Source: CAD feature listing. Evaluate the final solid. Frame: model axes, mm. A direction names the side the tool comes from. Round coordinates to 2 decimals unless told otherwise and drop trailing zeros. Loops run counter-clockwise (first coordinate to the right, second up) from the corner with the lowest first, then second, coordinate; pieces in that order, holes last. Notation, with made-up numbers: (2.5, 9.5) - (10.5, 9.5) arc R20 cw to (10.5, 19.5) - close; hole circle Ø7 at (70, 57). An arc over 180 degrees is marked (long way). One line per question, with ' | ' between items. Start each with the question number.
1. Ray query, line 1 (Z direction, x = -3.5, y = 5.75); line 2 (X direction, y = 0.75, z = -4.75); line 3 (X direction, y = -6.25, z = 1.5). Return the intervals inside material, ascending.
2. Pin query (flat end, axial travel): pin 1 (1.5 mm diameter, centred on x = 5.5, z = 1, fed in from -Y); pin 2 (2 mm diameter, centred on x = -8, z = 0.5, fed in from +Y). Return the tip coordinate at first contact, or that it passes through.
3. Cut plane B-B (z = 1.5). Return loops of the section in (x, y).
4. Cut plane C-C (y = 7.25). Return loops of the section in (x, z), then the cut area to 3 significant figures.
5. Access query for faces 1 (the flat face through (0, -7, 0)), 2 (the flat face through (-6, -4, 3.302)), 3 (the flat face through (-3.33, 5.81, 1.63)). Directions: +Z, -Z, +X, -X, +Y, -Y. A direction counts if a zero-diameter tool reaches every point of the face in a straight line with its end or side. Return the directions, or none.
6. Cut plane D-D (x = 6). Return loops of the section in (y, z).
7. Mould query, pull axis X, two halves, no side actions, for faces 4 (the flat face through (6, 4, 0)), 5 (the flat face through (2.487, 6.104, 1.628)), 6 (the flat face through (-6.53, -0.9, 1.63)), 7 (the flat face through (-3.366, -5.791, 1.628)). Classes: pulls with the +X half, pulls with the -X half, needs draft (parallel to the pull), parting line crosses it, or undercut.
```python
from build123d import *

# Parameters (mm, degrees)
F1_DEPTH    = 3.302
F2_DEPTH    = 6.35
F3_T1_DEPTH = 4.6338919233
F4_T1_DEPTH = 4.4582047696


# Not quite as in the source:
# - a fillet or chamfer that OpenCascade refuses, or shapes differently, is made with other operations: its cross-section is extruded or revolved along the edge and cut away or added


with BuildPart() as f1:
    # F0 (on Top) → F1 (new body)
    with BuildSketch(Plane.XY):
        with BuildLine():
            Line((0.8864303251, 2.1758656964), (4.1494522244, 10.1854037464))
            ThreePointArc((4.1494522244, 10.1854037464), (-0.7354841661, 10.9735803766), (-5.4715498037, 9.5405736717))
            Line((-5.4715498037, 9.5405736717), (-1.1688645655, 2.0381133132))
            ThreePointArc((-1.1688645655, 2.0381133132), (-0.157118442, 2.3442406116), (0.8864303251, 2.1758656964))
        make_face()
    extrude(amount=F1_DEPTH)



with BuildPart() as f1b:
    # F0 (on Top) → F1, piece 2 (new body)
    with BuildSketch(Plane.XY):
        with BuildLine():
            Line((-2.3275701308, -0.320261668), (-10.8955445044, -1.4991708351))
            ThreePointArc((-10.8955445044, -1.4991708351), (-9.1356572935, -6.1237381602), (-5.5266042645, -9.5087879639))
            Line((-5.5266042645, -9.5087879639), (-1.1806256223, -2.0313230639))
            ThreePointArc((-1.1806256223, -2.0313230639), (-1.9516127013, -1.3081888679), (-2.3275701308, -0.320261668))
        make_face()
    extrude(amount=F1_DEPTH)


with BuildPart() as f1c:
    # F0 (on Top) → F1, piece 3 (new body)
    with BuildSketch(Plane.XY):
        with BuildLine():
            ThreePointArc((6.74609228, -8.6862329113), (9.8711414597, -4.8498422164), (10.9981540682, -0.0317857078))
            Line((10.9981540682, -0.0317857078), (2.3494901878, -0.0067902494))
            ThreePointArc((2.3494901878, -0.0067902494), (2.1087311432, -1.0360517437), (1.4411398058, -1.8556040284))
            Line((1.4411398058, -1.8556040284), (6.74609228, -8.6862329113))
        make_face()
    extrude(amount=F1_DEPTH)


with BuildPart() as f1_1:
    add(f1.part)

    add(f1b.part)  # F2 merges F1b

    add(f1c.part)  # F2 merges F1c
    # F0 (on Top) → F2 (join)
    with BuildSketch(Plane.XY):
        with BuildLine():
            ThreePointArc((10.9981540682, -0.0317857078), (10.9981885171, -0.0158928705), (10.9982, 0))
            ThreePointArc((10.9982, 0), (9.1267986911, 6.136933183), (4.1494522244, 10.1854037464))
            Line((4.1494522244, 10.1854037464), (0.8864303251, 2.1758656964))
            ThreePointArc((0.8864303251, 2.1758656964), (1.9497202747, 1.3110076661), (2.3495, 0))
            ThreePointArc((2.3495, 0), (2.3494975469, -0.0033951282), (2.3494901878, -0.0067902494))
            Line((2.3494901878, -0.0067902494), (10.9981540682, -0.0317857078))
        make_face()
        with BuildLine():
            Line((0.8864303251, 2.1758656964), (4.1494522244, 10.1854037464))
            ThreePointArc((4.1494522244, 10.1854037464), (-0.7354841661, 10.9735803766), (-5.4715498037, 9.5405736717))
            Line((-5.4715498037, 9.5405736717), (-1.1688645655, 2.0381133132))
            ThreePointArc((-1.1688645655, 2.0381133132), (-0.157118442, 2.3442406116), (0.8864303251, 2.1758656964))
        make_face()
        with BuildLine():
            ThreePointArc((6.74609228, -8.6862329113), (9.8711414597, -4.8498422164), (10.9981540682, -0.0317857078))
            Line((10.9981540682, -0.0317857078), (2.3494901878, -0.0067902494))
            ThreePointArc((2.3494901878, -0.0067902494), (2.1087311432, -1.0360517437), (1.4411398058, -1.8556040284))
            Line((1.4411398058, -1.8556040284), (6.74609228, -8.6862329113))
        make_face()
        with BuildLine():
            Line((-1.1688645655, 2.0381133132), (-5.4715498037, 9.5405736717))
            ThreePointArc((-5.4715498037, 9.5405736717), (-9.8711414597, 4.8498422164), (-10.8955445044, -1.4991708351))
            Line((-10.8955445044, -1.4991708351), (-2.3275701308, -0.320261668))
            ThreePointArc((-2.3275701308, -0.320261668), (-2.1087311432, 1.0360517437), (-1.1688645655, 2.0381133132))
        make_face()
        with BuildLine():
            ThreePointArc((-5.5266042645, -9.5087879639), (0.7354841661, -10.9735803766), (6.74609228, -8.6862329113))
            Line((6.74609228, -8.6862329113), (1.4411398058, -1.8556040284))
            ThreePointArc((1.4411398058, -1.8556040284), (0.157118442, -2.3442406116), (-1.1806256223, -2.0313230639))
            Line((-1.1806256223, -2.0313230639), (-5.5266042645, -9.5087879639))
        make_face()
        with BuildLine():
            Line((-2.3275701308, -0.320261668), (-10.8955445044, -1.4991708351))
            ThreePointArc((-10.8955445044, -1.4991708351), (-9.1356572935, -6.1237381602), (-5.5266042645, -9.5087879639))
            Line((-5.5266042645, -9.5087879639), (-1.1806256223, -2.0313230639))
            ThreePointArc((-1.1806256223, -2.0313230639), (-1.9516127013, -1.3081888679), (-2.3275701308, -0.320261668))
        make_face()
    extrude(amount=-F2_DEPTH)

    # F3: fillet of radius 0.508 on 6 edges, made by hand

    # F3_s2 → F3_t1 (cut)
    with BuildSketch(Plane.XY):
        with BuildLine():
            ThreePointArc((3.9531481969, 9.7035483908), (3.9459668292, 10.1036299064), (3.6513440541, 10.3743958782))
            ThreePointArc((3.6513440541, 10.3743958782), (3.901542663, 10.2829163222), (4.1494522244, 10.1854037464))
            Line((4.1494522244, 10.1854037464), (3.9531481969, 9.7035483908))
        make_face()
        with BuildLine():
            ThreePointArc((10.9837113978, -0.5643466757), (10.8451967866, -0.1889395718), (10.4778487793, -0.0302819762))
            Line((10.4778487793, -0.0302819762), (10.9981540682, -0.0317857078))
            ThreePointArc((10.9981540682, -0.0317857078), (10.9941578867, -0.2981536556), (10.9837113978, -0.5643466757))
        make_face()
        with BuildLine():
            ThreePointArc((-5.212699429, 9.089224208), (-5.2589719244, 9.4866857122), (-5.0031171412, 9.7943464361))
            ThreePointArc((-5.0031171412, 9.7943464361), (-5.2388703034, 9.6702968509), (-5.4715498037, 9.5405736717))
            Line((-5.4715498037, 9.5405736717), (-5.212699429, 9.089224208))
        make_face()
        with BuildLine():
            ThreePointArc((7.1588183524, -8.3493546479), (6.7770167548, -8.4691224698), (6.4269453148, -8.2753009589))
            Line((6.4269453148, -8.2753009589), (6.74609228, -8.6862329113))
            ThreePointArc((6.74609228, -8.6862329113), (6.9544954285, -8.5202932212), (7.1588183524, -8.3493546479))
        make_face()
        with BuildLine():
            ThreePointArc((-5.9805942565, -9.2299997605), (-5.5862248623, -9.2977461404), (-5.2651493503, -9.0589422318))
            Line((-5.2651493503, -9.0589422318), (-5.5266042645, -9.5087879639))
            ThreePointArc((-5.5266042645, -9.5087879639), (-5.7552875833, -9.3721431953), (-5.9805942565, -9.2299997605))
        make_face()
        with BuildLine():
            ThreePointArc((-10.3800935118, -1.428247432), (-10.722983584, -1.6345074366), (-10.8101624065, -2.0250412303))
            ThreePointArc((-10.8101624065, -2.0250412303), (-10.8560380915, -1.762623101), (-10.8955445044, -1.4991708351))
            Line((-10.8955445044, -1.4991708351), (-10.3800935118, -1.428247432))
        make_face()
    extrude(amount=F3_T1_DEPTH, mode=Mode.SUBTRACT)

    # F4: fillet of radius 0.508 on 6 edges, made by hand

    # F4_s2 → F4_t1 (cut)
    with BuildSketch(Plane.XY):
        with BuildLine():
            ThreePointArc((-2.7857353042, -0.3833028373), (-2.4469491553, -0.4559663275), (-2.2335580647, -0.7289503561))
            ThreePointArc((-2.2335580647, -0.7289503561), (-2.2897006824, -0.5267077321), (-2.3275701308, -0.320261668))
            Line((-2.3275701308, -0.320261668), (-2.7857353042, -0.3833028373))
        make_face()
        with BuildLine():
            ThreePointArc((-1.5229431343, -1.7890764264), (-1.3515120564, -2.0901867434), (-1.4130231496, -2.4311741667))
            Line((-1.4130231496, -2.4311741667), (-1.1806256223, -2.0313230639))
            ThreePointArc((-1.1806256223, -2.0313230639), (-1.3572000088, -1.9178525455), (-1.5229431343, -1.7890764264))
        make_face()
        with BuildLine():
            ThreePointArc((-0.7879140674, 2.2134456561), (-1.1343987902, 2.215537146), (-1.3989470146, 2.439301027))
            Line((-1.3989470146, 2.439301027), (-1.1688645655, 2.0381133132))
            ThreePointArc((-1.1688645655, 2.0381133132), (-0.9823090207, 2.1342959584), (-0.7879140674, 2.2134456561))
        make_face()
        with BuildLine():
            ThreePointArc((0.4854895058, 2.2987932029), (0.8285961548, 2.3471032941), (1.0609176577, 2.6041689603))
            Line((1.0609176577, 2.6041689603), (0.8864303251, 2.1758656964))
            ThreePointArc((0.8864303251, 2.1758656964), (0.6887080648, 2.2462928241), (0.4854895058, 2.2987932029))
        make_face()
        with BuildLine():
            ThreePointArc((1.7248176465, -2.220866123), (1.6183530006, -1.8911369665), (1.7480685589, -1.5698428468))
            ThreePointArc((1.7480685589, -1.5698428468), (1.6009926176, -1.719585092), (1.4411398058, -1.8556040284))
            Line((1.4411398058, -1.8556040284), (1.7248176465, -2.220866123))
        make_face()
        with BuildLine():
            ThreePointArc((2.8119701642, -0.0081268603), (2.4859108466, -0.1253504027), (2.3108572018, -0.4243692296))
            ThreePointArc((2.3108572018, -0.4243692296), (2.3395090295, -0.2164434129), (2.3494901878, -0.0067902494))
            Line((2.3494901878, -0.0067902494), (2.8119701642, -0.0081268603))
        make_face()
    extrude(amount=F4_T1_DEPTH, mode=Mode.SUBTRACT)


solid = f1_1.part
```
Answers follow:
1) line 1: z = -6.35 to 0 | line 2: x = -10.97 to -2.23, 2.23 to 10.97 | line 3: x = -9.05 to -3.63, 4.85 to 9.05
2) pin 1: stops at y = -8.05 | pin 2: stops at y = 8.37
3) outline: (-10.81, -2.03) arc R11 ccw to (-5.98, -9.23) arc R0.51 ccw to (-5.27, -9.06) - (-1.41, -2.43) arc R0.51 ccw to (-1.52, -1.79) arc R2.35 cw to (-2.23, -0.73) arc R0.51 ccw to (-2.79, -0.38) - (-10.38, -1.43) arc R0.51 ccw to start; (-5.21, 9.09) - (-1.4, 2.44) arc R0.51 ccw to (-0.79, 2.21) arc R2.35 cw to (0.49, 2.3) arc R0.51 ccw to (1.06, 2.6) - (3.95, 9.7) arc R0.51 ccw to (3.65, 10.37) arc R11 ccw to (-5, 9.79) arc R0.51 ccw to start; (1.72, -2.22) - (6.43, -8.28) arc R0.51 ccw to (7.16, -8.35) arc R11 ccw to (10.98, -0.56) arc R0.51 ccw to (10.48, -0.03) - (2.81, -0.01) arc R0.51 ccw to (2.31, -0.42) arc R2.35 cw to (1.75, -1.57) arc R0.51 ccw to start
4) outline: (-8.27, -6.35) - (8.27, -6.35) - (8.27, 0) - (2.95, 0) - (2.95, 3.3) - (-4.16, 3.3) - (-4.16, 0) - (-8.27, 0) - close | area: 129 mm2
5) face 1: +Z, -Y | face 2: +Z, +X, -X, +Y, -Y | face 3: +Z, -X
6) outline: (-9.22, -6.35) - (9.22, -6.35) - (9.22, 0) - (-0.02, 0) - (-0.02, 3.3) - (-7.73, 3.3) - (-7.73, 0) - (-9.22, 0) - close
7) face 4: needs draft | face 5: pulls with the +X half | face 6: pulls with the -X half | face 7: undercut
